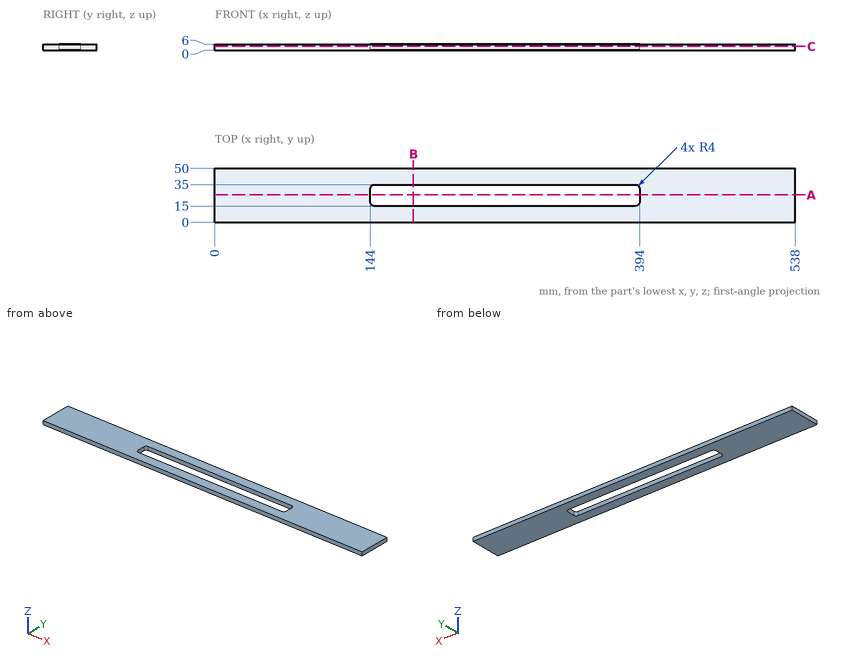
Answer from the drawing. Dimensions are ordinates in mm from the lowest x, y and z of the part. Give positions to 0.01 mm unless a question says otherwise; leave off trailing zeros. Write each loop counter-clockwise with the first axis right and the second up, starting at its lowest first coordinate (ties: lowest second). Pieces come first, ordered by that corner, then holes. Notation, with made-up numbers: (28, 11) -> (78, 11) arc R18 cw to (78, 26) -> close; hole circle Ø11 at (73, 31.25). An arc over 180 degrees is marked (long way). Use a Markdown table: item, result.
(1) Section C-C, the plane z = 3.85 is taken. Determine the outline of the cut face in (x, y).
Return value:
| item | result |
|---|---|
| outline | (0, 0) -> (538, 0) -> (538, 50) -> (0, 50) -> close; hole (144, 19) arc R4 ccw to (148, 15) -> (390, 15) arc R4 ccw to (394, 19) -> (394, 31) arc R4 ccw to (390, 35) -> (148, 35) arc R4 ccw to (144, 31) -> close |
(2) Section B-B, the plane x = 184 is taken. Determine the outline of the cut face in (y, z), then the cut area to 3 significant figures.
Return value:
| item | result |
|---|---|
| outline | (0, 0) -> (15, 0) -> (15, 6) -> (0, 6) -> close; (35, 0) -> (50, 0) -> (50, 6) -> (35, 6) -> close |
| area | 180 mm2 |
(3) Find the intervals of material crossed by probe 1 along Y at (x, z) = (294.5, 3.65); probe 2 along X at (y, z) = (27, 3.4); probe 3 along X at (y, z) = (16, 4.75), in increasing order. Write a range as from..to.
Return value:
| item | result |
|---|---|
| probe 1 | 0..15, 35..50 |
| probe 2 | 0..144, 394..538 |
| probe 3 | 0..145.35, 392.65..538 |
(4) Section A-A, the plane y = 25.5 is taken. Determine the outline of the cut face in (x, z).
Return value:
| item | result |
|---|---|
| outline | (0, 0) -> (144, 0) -> (144, 6) -> (0, 6) -> close; (394, 0) -> (538, 0) -> (538, 6) -> (394, 6) -> close |
